from build123d import *

# Parameters (mm, degrees)
F1_DEPTH = 5


with BuildPart() as f1:
    # F0 (on Top) → F1 (new body)
    with BuildSketch(Plane.XY):
        with BuildLine():
            Line((-11.91868, 14), (-20, 14))
            Line((-20, 14), (-20, 9))
            Line((-20, 9), (-10, 9))
            Line((-10, 9), (-10, 5))
            ThreePointArc((-10, 5), (-8.535534, 1.464466), (-5, 0))
            Line((-5, 0), (0, 0))
            Line((0, 0), (70, 0))
            ThreePointArc((70, 0), (68.535534, 3.535534), (65, 5))
            Line((65, 5), (1.91868, 5))
            ThreePointArc((1.91868, 5), (0.127361, 5.331898), (-1.426144, 6.283529))
            Line((-1.426144, 6.283529), (-8.573856, 12.716471))
            ThreePointArc((-8.573856, 12.716471), (-10.127361, 13.668102), (-11.91868, 14))
        make_face()
    extrude(amount=F1_DEPTH)


solid = f1.part
Check sheet for the modelled part. Datum: model origin and axes. Units: mm. A direction names the side the tool comes from. Give positions to 0.01 mm unless a question says otherwise; leave off trailing zeros. Write each loop counter-clockwise with the first axis right and the second up, starting at its lowest first coordinate (ties: lowest second). Pieces come first, ordered by that corner, then holes. Notation, with made-up numbers: (57, 74) -> (67, 74) arc R26 cw to (67, 110) -> close; hole circle Ø7 at (89.25, -11). An arc over 180 degrees is marked (long way). One line per item, written item: value. Start each with the question number.
Item 1: Material ranges on probe 1 along Y at (x, z) = (23.5, 0.5); probe 2 along X at (y, z) = (8.75, 2.7); probe 3 along X at (y, z) = (8.25, 1.55), recorded low to high. Write a range as from..to.
Item 2: Tool access check on faces 1 (the flat face through (34, 5, 2)), 2 (the flat face through (-10, 7, 2)), 3 (the flat face through (32, 0, 2)). Record the directions out of +Z, -Z, +X, -X, +Y, -Y that give a thin tool (end or side, any length) a straight path to the whole face; none if there is none.
Item 3: Section check A-A on z = 1.8. Record the cut outline in (x, y).
Item 4: Section check B-B on x = 11. Record the cut outline in (y, z), then the cut area to 3 significant figures.
Item 5: Section check C-C on y = 10.5. Record the cut outline in (x, z), then the cut area to 3 significant figures.
Item 6: Gauge pin test, flat ends, axial feed: pin 1 (2.5 mm diameter, centred on x = -15.5, z = 2.5, fed in from -Y); pin 2 (2 mm diameter, centred on x = 51, z = 1.5, fed in from +Y); pin 3 (2 mm diameter, centred on y = 6.5, z = 1.5, fed in from -X). Record the tip position at first contact, or that the pin passes through.
Results list:
1. probe 1: 0..5
1. probe 2: -10..-4.17
1. probe 3: -10..-3.61
2. face 1: +Z, -Z, +X, +Y
2. face 2: +Z, -Z, -X, -Y
2. face 3: +Z, -Z, +X, -X, -Y
3. outline: (-20, 9) -> (-10, 9) -> (-10, 5) arc R5 ccw to (-5, 0) -> (70, 0) arc R5 ccw to (65, 5) -> (1.92, 5) arc R5 cw to (-1.43, 6.28) -> (-8.57, 12.72) arc R5 ccw to (-11.92, 14) -> (-20, 14) -> close
4. outline: (0, 0) -> (5, 0) -> (5, 5) -> (0, 5) -> close
4. area: 25.0 mm²
5. outline: (-20, 0) -> (-6.11, 0) -> (-6.11, 5) -> (-20, 5) -> close
5. area: 69.4 mm²
6. pin 1: y = 9
6. pin 2: y = 5
6. pin 3: x = -10
